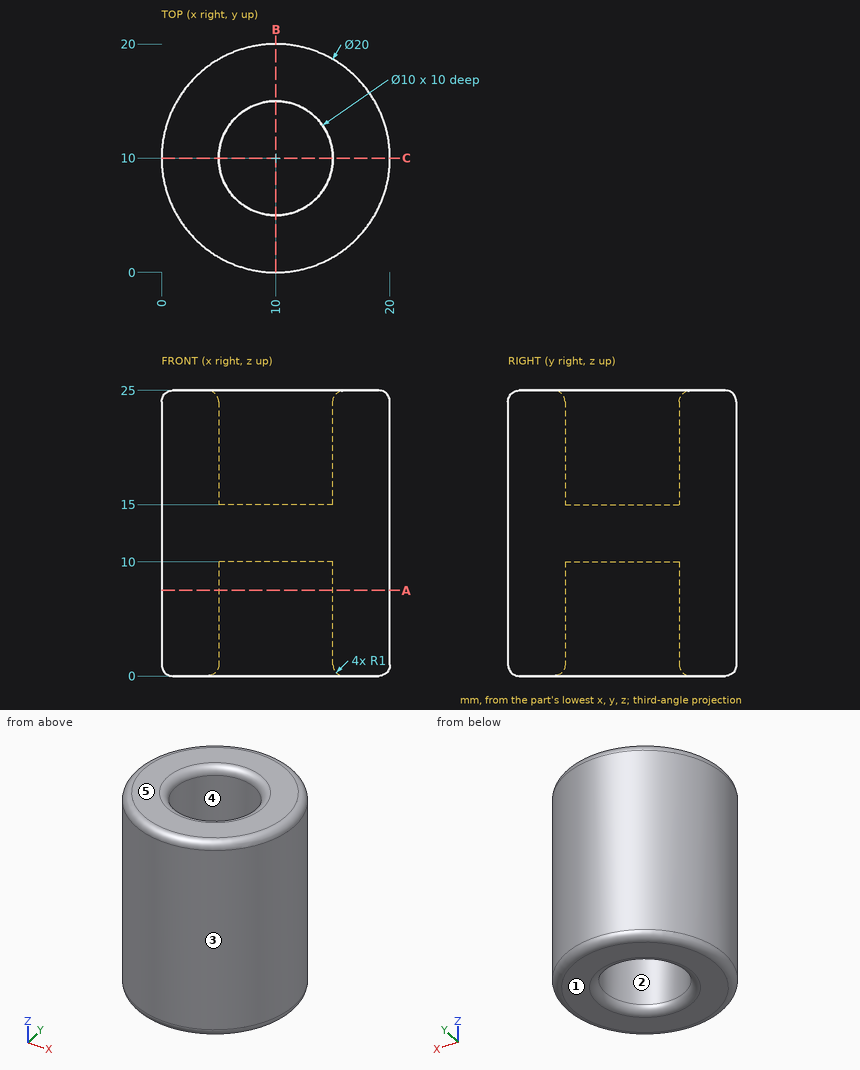
Could you check a few things on this drawing? It's one solid part, dimensions in mm from its lowest x, y, z. A direction names the side the tool comes from. Round coordinates to 2 decimals unless told otherwise and drop trailing zeros. Write each loop counter-clockwise with the first axis right and the second up, starting at its lowest first coordinate (ties: lowest second). Pieces come first, ordered by that corner, then holes. Notation, with made-up numbers: (61.5, -8.5) -> (90.5, -8.5) arc R13 cw to (90.5, 16.5) -> close; hole circle Ø7 at (-35.75, -24.5). An arc over 180 degrees is marked (long way). One line per question, with ' | ' between items. Start each with the question number.
1) I'm going to push flat-ended pins straight in: P1, Ø4, axis at x = 6.5, z = 21, coming from the +Y side; P2, Ø8, axis at x = 10, y = 10, coming from the +Z side; P3, Ø4, axis at x = 14.5, z = 20.5, coming from the -Y side. Where does each tip first touch, or does it pass through?
2) Suppose I cut it at A-A on z = 7.5. Write out the boundary of the cut face in (x, y).
3) If we mould it in two halves opening along X, with no side actions, what happens to the marked faces 1, 2 and 3? For each: released by +X, released by -X, zero draft, split by the parting line, or undercut.
4) On a 3-axis mill with a long thin cutter (end or side, diameter ignored), from which of +Z, -Z, +X, -X, +Y, -Y can I reach the whole of each face in a straight line? I mean the marked faces 4 and 5. Say none if no direction works.
5) Suppose I cut it at B-B on x = 10. Write out the boundary of the cut face in (y, z), then the cut area to 3 significant figures.
6) I need wall thicknesses on line 1 (Y direction, x = 10, z = 22); line 2 (X direction, y = 13.25, z = 7.25); line 3 (Z direction, x = 7.75, y = 11). Which ranges of each line are inside material? Lowest first, please. Write a range as [from, to].
Return value:
1) P1: stops at y = 19.89 | P2: stops at z = 15 | P3: stops at y = 0.32
2) outline: circle Ø20 at (10, 10); hole circle Ø10 at (10, 10)
3) face 1: zero draft | face 2: undercut | face 3: split by the parting line
4) face 4: +Z | face 5: +Z, +X, -X, +Y, -Y
5) outline: (0, 1) arc R1 ccw to (1, 0) -> (4, 0) arc R1 ccw to (5, 1) -> (5, 10) -> (15, 10) -> (15, 1) arc R1 ccw to (16, 0) -> (19, 0) arc R1 ccw to (20, 1) -> (20, 24) arc R1 ccw to (19, 25) -> (16, 25) arc R1 ccw to (15, 24) -> (15, 15) -> (5, 15) -> (5, 24) arc R1 ccw to (4, 25) -> (1, 25) arc R1 ccw to (0, 24) -> close | area: 298 mm2
6) line 1: y = [0, 5], [15, 20] | line 2: x = [0.54, 6.2], [13.8, 19.46] | line 3: z = [10, 15]
